from build123d import *

# Parameters (mm, degrees)
F0_W     = 33.5
F0_H     = 50.8
F1_DEPTH = 5.9
F3_DEPTH = 0.1


with BuildPart() as f1:
    # F0 (on Top) → F1 (new body)
    with BuildSketch(Plane.XY):
        Rectangle(F0_W, F0_H)
    extrude(amount=F1_DEPTH)

    # F2 (on face) → F3 (cut)
    with BuildSketch(Plane(origin=(0, 0, 0), x_dir=(1, 0, 0), z_dir=(0, 0, -1))):
        with BuildLine():
            ThreePointArc((0.5, -23.4), (-0.353553, -23.046447), (0, -23.9))
            ThreePointArc((0, -23.9), (0.353553, -23.753553), (0.5, -23.4))
        make_face()
    extrude(amount=-F3_DEPTH, mode=Mode.SUBTRACT)


solid = f1.part
Model file for the job. Use its own axes, mm. Give positions to 0.01 mm unless a question says otherwise; leave off trailing zeros. One line per item, written item: value.
Item 1: Wall check: line 1 (Y direction, x = 0, z = 0.05). Give the ranges that are in metal, low to high.
Response values:
line 1: -25.4 to 22.9, 23.9 to 25.4
Item 2: Two-plate mould, pull along Y, no slides. Class faces 1 (the flat face through (-16.75, 0, 3)), 2 (the flat face through (0, 25.4, 3)), 3 (the flat face through (0, 23.4, 0.1)), 4 (the flat face through (0, -25.4, 3)): released by +Y, released by -Y, zero draft, split by the parting line, or undercut.
Response values:
face 1: zero draft
face 2: released by +Y
face 3: undercut
face 4: released by -Y
Item 3: Pin check, flat tip, straight feed: pin 1 Ø1.1 at (x, y) = (0, 23.5) entering from -Z. Stop position of the tip, or through.
Response values:
pin 1: z = 0
